Answer from the drawing. Dimensions are ordinates in mm from the lowest x, y and z of the part. A direction names the side the tool comes from. Give positions to 0.01 mm unless a question says otherwise; leave off trailing zeros. Order: outer loops, then holes, each group sorted by start corner. A loop starts at its lowest first (then second) coordinate and runs counter-clockwise, first axis right, second up. Notation, with made-up numbers: M 2.5,48.25 L 56.5,48.25 A25 ccw 56.5,64.25 Z; hole C 37,-23 d2. An arc over 180 degrees is marked long. One line per item, written item: value.
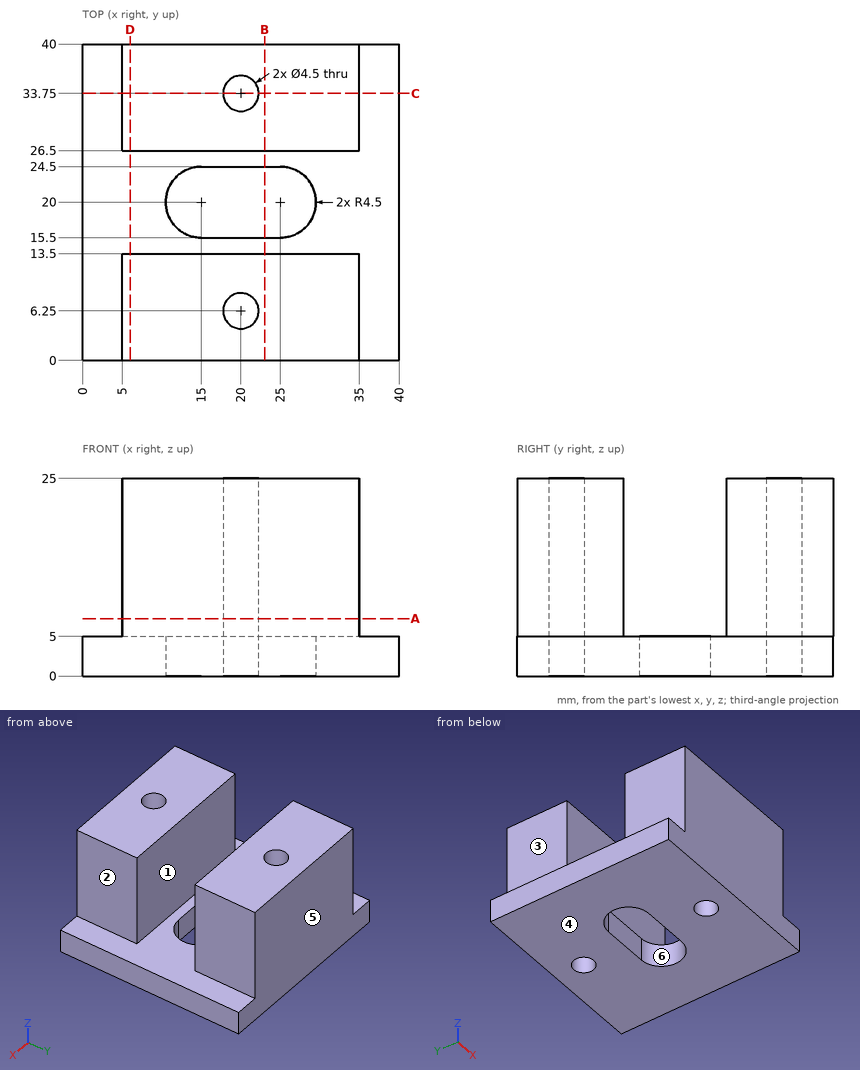
(1) Section B-B, the plane x = 23 is taken. Give the vertices of the cut face in (y, z), then the cut area to 3 significant figures.
Findings:
outline: M 0,0 L 15.5,0 L 15.5,5 L 13.5,5 L 13.5,25 L 0,25 Z; M 24.5,0 L 40,0 L 40,25 L 26.5,25 L 26.5,5 L 24.5,5 Z
area: 695 mm^2
(2) Given P1, Ø11, axis at y = 4.5, z = 18, coming from the +X side; P2, Ø4, axis at y = 8, z = 12.5, coming from the -X side, each flat-ended and moving along its own axis, determine where each tip first touches the part or whether it passes through.
Findings:
P1: stops at x = 35
P2: stops at x = 5
(3) Section A-A, the plane z = 7.25 is taken. Give the vertices of the cut face in (x, y).
Findings:
outline: M 5,0 L 35,0 L 35,13.5 L 5,13.5 Z; M 5,26.5 L 35,26.5 L 35,40 L 5,40 Z; hole C 20,6.25 d4.5; hole C 20,33.75 d4.5
(4) Find the intervals of material crossed by probe 1 along Y at (x, z) = (20, 18); probe 2 along Y at (x, z) = (25, 22); probe 3 along Z at (x, y) = (2.5, 18), in increasing order. Write a range as from..to.
Findings:
probe 1: y = 0..4, 8.5..13.5, 26.5..31.5, 36..40
probe 2: y = 0..13.5, 26.5..40
probe 3: z = 0..5
(5) Section C-C, the plane y = 33.75 is taken. Give the vertices of the cut face in (x, z), then the cut area to 4 significant figures.
Findings:
outline: M 0,0 L 17.75,0 L 17.75,25 L 5,25 L 5,5 L 0,5 Z; M 22.25,0 L 40,0 L 40,5 L 35,5 L 35,25 L 22.25,25 Z
area: 687.5 mm^2
(6) Section D-D, the plane x = 6 is taken. Give the vertices of the cut face in (y, z).
Findings:
outline: M 0,0 L 40,0 L 40,25 L 26.5,25 L 26.5,5 L 13.5,5 L 13.5,25 L 0,25 Z
(7) Which of the six approach directions +Z, -Z, +X, -X, +Y, -Y give full straight-line access (tool end or side, diameter ignored) to the marked faces 1, 2 and 3?
Findings:
face 1: +Z, +X, -X
face 2: +Z, +X, +Y, -Y
face 3: +Z, -X, +Y, -Y
(8) Determine the mould class of the marked faces 4, 5 and 6 for opening direction Y: pulls with the +Y half, pulls with the -Y half, needs draft (parallel to the pull), parting line crosses it, or undercut.
Findings:
face 4: needs draft
face 5: pulls with the +Y half
face 6: undercut
